Solid Edge part; units mm, degrees
sketch "Sketch1" plane through (0, 0, 0) normal (0, 0, 1) x (1, 0, 0)
  line L0 (-142.255, -41.75) -> (142.255, -41.75)
  line L1 (142.255, -41.75) -> (142.255, 41.75)
  line L2 (142.255, 41.75) -> (-142.255, 41.75)
  line L3 (-142.255, 41.75) -> (-142.255, -41.75)
extrude "Protrusion1" add sketch "Sketch1" against normal blind 20
sketch "Sketch2" plane through (0, 0, 0) normal (0, 0, 1) x (0, 1, 0)
  circle A0 centre (-6.75, -81.075) radius 6.5
  circle A1 centre (-11.75, -177.075) radius 60
extrude "ExtrudedCutout_1" cut sketch "Sketch2" against normal blind 20
fillet "Round_2" radius 3 1 edges at (125.1135, -41.75, -10)
fillet "Round_3" radius 5 1 edges at (142.255, 41.75, -10)
Input: part model. Units: mm. Frame: model coordinates. Round coordinates to 2 decimals unless told otherwise and drop trailing zeros. Order: outer loops, then holes, each group sorted by start corner. A loop starts at its lowest first (then second) coordinate and runs counter-clockwise, first axis right, second up. Notation, with made-up numbers: (74.25, 67.5) - (80.25, 67.5) arc R25 ccw to (80.25, 81.5) - close; hole circle Ø7 at (41, 41.5). An arc over 180 degrees is marked (long way). Answer in a Markdown table with one row per item.
Item 1: Section query A-A (y = -5.5). Return the cut outline in (x, z) (3 decimals).
Model answer:
| item | result |
|---|---|
| outline | (-142.255, -20) - (74.696, -20) - (74.696, 0) - (-142.255, 0) - close; (87.454, -20) - (117.401, -20) - (117.401, 0) - (87.454, 0) - close |
Item 2: Section query B-B (z = -7.75). Return the cut outline in (x, y) (3 decimals), then the cut area to 3 significant figures.
Model answer:
| item | result |
|---|---|
| outline | (-142.255, -41.75) - (120.154, -41.75) arc R3 ccw to (122.865, -37.464) arc R60 cw to (142.255, 37.113) arc R5 ccw to (137.268, 41.75) - (-142.255, 41.75) - close; hole circle Ø13 at (81.075, -6.75) |
| area | 22,100 mm² |
Item 3: Pin query (flat end, axial travel): pin 1 (3 mm diameter, centred on y = 6.5, z = -6.5, fed in from +X). Return the tip coordinate at first contact, or that it passes through.
Model answer:
| item | result |
|---|---|
| pin 1 | stops at x = 120.42 |
Item 4: Section query C-C (y = -29.5). Return the cut outline in (x, z) (3 decimals), then the cut area to 3 significant figures.
Model answer:
| item | result |
|---|---|
| outline | (-142.255, -20) - (119.761, -20) - (119.761, 0) - (-142.255, 0) - close |
| area | 5,240 mm² |
Item 5: Mould query, pull axis Y, two halves, no side actions, for faces 1 (the cylindrical face through (79.12, -0.55, -9.86)), 2 (the flat face through (-2, 1, -20)), 3 (the flat face through (-1, 41.75, -10)), 4 (the cylindrical face through (119.156, 3.914, -9.86)). Classes: released by +Y, released by -Y, zero draft, split by the parting line, or undercut.
Model answer:
| item | result |
|---|---|
| face 1 | undercut |
| face 2 | zero draft |
| face 3 | released by +Y |
| face 4 | undercut |
Item 6: Line query: line 1 (X direction, y = -6.75, z = -14.5) (3 decimals); line 2 (Y direction, x = 77, z = -9.5); line 3 (X direction, y = -35.5, z = -18) (3 decimals). Output: solid intervals per line, ascending.
Model answer:
| item | result |
|---|---|
| line 1 | x = -142.255 to 74.575, 87.575 to 117.284 |
| line 2 | y = -41.75 to -11.81, -1.69 to 41.75 |
| line 3 | x = -142.255 to 121.976 |
